Geometry: final body of the model. Coordinates: model frame, mm. A direction names the side the tool comes from. Round coordinates to 2 decimals unless told otherwise and drop trailing zeros. Write each loop counter-clockwise with the first axis right and the second up, starting at its lowest first coordinate (ties: lowest second). Pieces come first, ordered by that corner, then holes. Notation, with made-up numbers: (80, 64.5) -> (87, 64.5) arc R23 ccw to (87, 84.5) -> close; hole circle Ø1 at (-11, 20). An arc over 180 degrees is marked (long way). Use one line per item in the form item = value. Start each with the question number.
1. Reachability of faces 1 (the face through (4.375, -2.5, 2.2)), 2 (the face through (0.106, 2.603, 4.483)) from +Z, -Z, +X, -X, +Y, -Y: full face, straight path, thin tool, end or side. Return the list, or none.
2. Line query: L1, parallel to X at y = -2, z = 3.5 (3 decimals); L2, parallel to Z at x = 20.5, y = -1.5; L3, parallel to Y at x = 2.75, z = 2.5. Output: solid intervals per line, ascending.
3. Cut plane A-A, the plane x = 3.5. Return the cut outline in (y, z).
4. Cut plane B-B, the plane x = 22.25. Return the cut outline in (y, z).
5. Pin query (flat end, axial travel): pin 1 Ø6 at (x, z) = (22, -2) entering from +Y. Return the tip coordinate at first contact, or that it passes through.
```python
from build123d import *

# Parameters (mm, degrees)
BASEHEAD_DEPTH = 4.375


# Read off the part's stored shape, not the designer's step: HeadChamfer
with BuildPart() as part:
    # Sketch1 → BaseHead (new body)
    with BuildSketch(Plane(origin=(0, 0, 0), x_dir=(0, 0, -1), z_dir=(1, 0, 0))):
        Polygon((5, 2.886751346), (5, -2.886751346), (0, -5.773502692), (-5, -2.886751346), (-5, 2.886751346), (0, 5.773502692), align=None)
    extrude(amount=BASEHEAD_DEPTH)

    # HeadChamfer outline → HeadChamfer (revolve, cut)
    with BuildSketch(Plane.YX):
        Polygon((5.773502688, 0.446581985), (4.999998827, -6.77e-07), (5.773502692, -8.45e-07), align=None)
    revolve(axis=Axis((0, 0, 0), (1, 0, 0)), mode=Mode.SUBTRACT)

    # HeadChamfer 2 outline → HeadChamfer 2 (revolve)
    with BuildSketch(Plane.YX):
        Polygon((3, 4.375), (3, 23.8205), (2.4455, 24.375), (0, 24.375), (0, 4.375), align=None)
    revolve(axis=Axis((0, 0, 0), (1, 0, 0)))


solid = part.part
```
Outcome:
q1.face_1 = +X
q1.face_2 = +Z, -X, +Y
q2.L1 = 0 to 4.375
q2.L2 = -2.6 to 2.6
q2.L3 = -4.33 to 4.33
q3.outline = (-5.77, 0) -> (-2.89, -5) -> (2.89, -5) -> (5.77, 0) -> (2.89, 5) -> (-2.89, 5) -> close
q4.outline = circle Ø6 at (0, 0)
q5.pin_1 = 3
